Work out the finished part from the listing and answer in its coordinate system (mm). A direction names the side the tool comes from. Coordinates: 2 decimals unless noted, no trailing zeros. Loops run counter-clockwise (first coordinate to the right, second up) from the corner with the lowest first, then second, coordinate; pieces in that order, holes last. Notation, with made-up numbers: M -3,61.25 L 47,61.25 A18 ccw 47,73.25 Z; hole C 37.5,-0.75 d4. An arc over 180 degrees is marked long. Write each question's results on one line, items separated by ' | '.
```python
from build123d import *

# Parameters (mm, degrees)
F0_W     = 4.0655732155
F0_H     = 10
F0_W_2   = 10
F0_H_2   = 4.0655732155
F1_DEPTH = 60
F2_DEPTH = 10
F3_DEPTH = 1


with BuildPart() as f1:
    # F0 (on Top) → F1 (new body)
    with BuildSketch(Plane.XY):
        Polygon((-81.7574552458, 91.9649731191), (-85.0374214202, 91.9649731191), (-85.0374214202, 87.5400633349), (-85.0374214202, 55.211449102), (-85.0374214202, -53.3124324366), (-85.0374214202, -86.6156537372), (-85.0374214202, -90.0350268809), (-80.8175235253, -90.0350268809), (-48.580678454, -90.0350268809), (96.9625785798, -90.0350268809), (96.9625785798, 91.9649731191), align=None)
        Polygon((-33.0721171855, -88.258663221), (-43.0721171855, -88.258663221), (-48.580678454, -88.258663221), (-64.0721171855, -88.258663221), (-64.0721171855, -84.1930900056), (-43.0721171855, -84.1930900056), (-33.0721171855, -84.1930900056), (-33.0721171855, -84.127867623), (-12.0721171855, -84.127867623), (-12.0721171855, -88.258663221), align=None, mode=Mode.SUBTRACT)
        Polygon((-79.1745140415, -38.1238959565), (-79.1745140415, -48.1238959565), (-79.1745140415, -53.3124324366), (-79.1745140415, -69.1238959565), (-83.240087257, -69.1238959565), (-83.240087257, -53.3124324366), (-83.240087257, -48.1238959565), (-83.240087257, -38.1238959565), (-83.3053096395, -38.1238959565), (-83.3053096395, -17.1238959565), (-79.1745140415, -17.1238959565), align=None, mode=Mode.SUBTRACT)
        Polygon((44.9625785798, -83.9851424098), (54.9625785798, -83.9851424098), (60.1511150599, -83.9851424098), (75.9625785798, -83.9851424098), (75.9625785798, -88.0507156253), (60.1511150599, -88.0507156253), (54.9625785798, -88.0507156253), (44.9625785798, -88.0507156253), (44.9625785798, -88.1159380078), (23.9625785798, -88.1159380078), (23.9625785798, -83.9851424098), align=None, mode=Mode.SUBTRACT)
        Polygon((94.8935046063, -37.9912286836), (94.8935046063, -47.9912286836), (94.8935046063, -53.1797651637), (94.8935046063, -68.9912286836), (90.8279313908, -68.9912286836), (90.8279313908, -53.1797651637), (90.8279313908, -47.9912286836), (90.8279313908, -37.9912286836), (90.7627090082, -37.9912286836), (90.7627090082, -16.9912286836), (94.8935046063, -16.9912286836), align=None, mode=Mode.SUBTRACT)
        Polygon((-83.4004647296, 40.0229126219), (-83.4004647296, 50.0229126219), (-83.4004647296, 55.211449102), (-83.4004647296, 71.0229126219), (-79.3348915141, 71.0229126219), (-79.3348915141, 55.211449102), (-79.3348915141, 50.0229126219), (-79.3348915141, 40.0229126219), (-79.2696691316, 40.0229126219), (-79.2696691316, 19.0229126219), (-83.4004647296, 19.0229126219), align=None, mode=Mode.SUBTRACT)
        Polygon((-77.3635556847, 55.211449102), (-77.3635556847, 83.9649731191), (-48.3621415186, 83.9649731191), (61.3571461726, 83.9649731191), (88.6364443153, 83.9649731191), (88.6364443153, -82.0350268809), (-77.3635556847, -82.0350268809), (-77.3635556847, -53.3124324366), align=None, mode=Mode.SUBTRACT)
        Polygon((-33.1736050386, 85.8970538511), (-43.1736050386, 85.8970538511), (-48.3621415186, 85.8970538511), (-64.1736050386, 85.8970538511), (-64.1736050386, 89.9626270666), (-48.3621415186, 89.9626270666), (-43.1736050386, 89.9626270666), (-33.1736050386, 89.9626270666), (-33.1736050386, 90.0278494491), (-12.1736050386, 90.0278494491), (-12.1736050386, 85.8970538511), align=None, mode=Mode.SUBTRACT)
        Polygon((90.7789625961, 39.9640733615), (90.7789625961, 49.9640733615), (90.7789625961, 55.1526098416), (90.7789625961, 70.9640733615), (94.8445358116, 70.9640733615), (94.8445358116, 55.1526098416), (94.8445358116, 49.9640733615), (94.8445358116, 39.9640733615), (94.9097581941, 39.9640733615), (94.9097581941, 18.9640733615), (90.7789625961, 18.9640733615), align=None, mode=Mode.SUBTRACT)
        Polygon((44.9113614697, 89.7324799762), (54.9113614697, 89.7324799762), (61.3571461726, 89.7324799762), (75.9113614697, 89.7324799762), (75.9113614697, 85.6669067607), (61.3571461726, 85.6669067607), (54.9113614697, 85.6669067607), (44.9113614697, 85.6669067607), (44.9113614697, 85.6016843782), (23.9113614697, 85.6016843782), (23.9113614697, 89.7324799762), align=None, mode=Mode.SUBTRACT)
        Polygon((-79.3348915141, 40.0229126219), (-83.4004647296, 40.0229126219), (-83.4004647296, 19.0229126219), (-79.2696691316, 19.0229126219), (-79.2696691316, 40.0229126219), align=None)
        with Locations((-81.3676781219, 45.0229126219)):
            Rectangle(F0_W, F0_H)
        Polygon((-83.4004647296, 55.211449102), (-83.4004647296, 50.0229126219), (-79.3348915141, 50.0229126219), (-79.3348915141, 55.211449102), (-79.3348915141, 71.0229126219), (-83.4004647296, 71.0229126219), align=None)
        Polygon((-48.3621415186, 85.8970538511), (-43.1736050386, 85.8970538511), (-43.1736050386, 89.9626270666), (-48.3621415186, 89.9626270666), (-64.1736050386, 89.9626270666), (-64.1736050386, 85.8970538511), align=None)
        with Locations((-38.1736050386, 87.9298404588)):
            Rectangle(F0_W_2, F0_H_2)
        Polygon((-33.1736050386, 89.9626270666), (-33.1736050386, 85.8970538511), (-12.1736050386, 85.8970538511), (-12.1736050386, 90.0278494491), (-33.1736050386, 90.0278494491), align=None)
        Polygon((44.9113614697, 85.6669067607), (44.9113614697, 89.7324799762), (23.9113614697, 89.7324799762), (23.9113614697, 85.6016843782), (44.9113614697, 85.6016843782), align=None)
        with Locations((49.9113614697, 87.6996933685)):
            Rectangle(F0_W_2, F0_H_2)
        Polygon((61.3571461726, 89.7324799762), (54.9113614697, 89.7324799762), (54.9113614697, 85.6669067607), (61.3571461726, 85.6669067607), (75.9113614697, 85.6669067607), (75.9113614697, 89.7324799762), align=None)
        Polygon((90.7789625961, 55.1526098416), (90.7789625961, 49.9640733615), (94.8445358116, 49.9640733615), (94.8445358116, 55.1526098416), (94.8445358116, 70.9640733615), (90.7789625961, 70.9640733615), align=None)
        with Locations((92.8117492038, 44.9640733615)):
            Rectangle(F0_W, F0_H)
        Polygon((94.8445358116, 39.9640733615), (90.7789625961, 39.9640733615), (90.7789625961, 18.9640733615), (94.9097581941, 18.9640733615), (94.9097581941, 39.9640733615), align=None)
        Polygon((90.8279313908, -37.9912286836), (94.8935046063, -37.9912286836), (94.8935046063, -16.9912286836), (90.7627090082, -16.9912286836), (90.7627090082, -37.9912286836), align=None)
        with Locations((92.8607179985, -42.9912286836)):
            Rectangle(F0_W, F0_H)
        Polygon((94.8935046063, -53.1797651637), (94.8935046063, -47.9912286836), (90.8279313908, -47.9912286836), (90.8279313908, -53.1797651637), (90.8279313908, -68.9912286836), (94.8935046063, -68.9912286836), align=None)
        Polygon((60.1511150599, -83.9851424098), (54.9625785798, -83.9851424098), (54.9625785798, -88.0507156253), (60.1511150599, -88.0507156253), (75.9625785798, -88.0507156253), (75.9625785798, -83.9851424098), align=None)
        with Locations((49.9625785798, -86.0179290175)):
            Rectangle(F0_W_2, F0_H_2)
        Polygon((44.9625785798, -88.0507156253), (44.9625785798, -83.9851424098), (23.9625785798, -83.9851424098), (23.9625785798, -88.1159380078), (44.9625785798, -88.1159380078), align=None)
        Polygon((-33.0721171855, -84.1930900056), (-33.0721171855, -88.258663221), (-12.0721171855, -88.258663221), (-12.0721171855, -84.127867623), (-33.0721171855, -84.127867623), align=None)
        with Locations((-38.0721171855, -86.2258766133)):
            Rectangle(F0_W_2, F0_H_2)
        Polygon((-48.580678454, -88.258663221), (-43.0721171855, -88.258663221), (-43.0721171855, -84.1930900056), (-64.0721171855, -84.1930900056), (-64.0721171855, -88.258663221), align=None)
        Polygon((-79.1745140415, -53.3124324366), (-79.1745140415, -48.1238959565), (-83.240087257, -48.1238959565), (-83.240087257, -53.3124324366), (-83.240087257, -69.1238959565), (-79.1745140415, -69.1238959565), align=None)
        with Locations((-81.2073006492, -43.1238959565)):
            Rectangle(F0_W, F0_H)
        Polygon((-83.240087257, -38.1238959565), (-79.1745140415, -38.1238959565), (-79.1745140415, -17.1238959565), (-83.3053096395, -17.1238959565), (-83.3053096395, -38.1238959565), align=None)
    extrude(amount=-F1_DEPTH)

    # F0 (on Top) → F2 (cut)
    with BuildSketch(Plane.XY):
        Polygon((-83.4004647296, 55.211449102), (-83.4004647296, 50.0229126219), (-79.3348915141, 50.0229126219), (-79.3348915141, 55.211449102), (-79.3348915141, 71.0229126219), (-83.4004647296, 71.0229126219), align=None)
        Polygon((-79.3348915141, 40.0229126219), (-83.4004647296, 40.0229126219), (-83.4004647296, 19.0229126219), (-79.2696691316, 19.0229126219), (-79.2696691316, 40.0229126219), align=None)
        Polygon((90.7789625961, 55.1526098416), (90.7789625961, 49.9640733615), (94.8445358116, 49.9640733615), (94.8445358116, 55.1526098416), (94.8445358116, 70.9640733615), (90.7789625961, 70.9640733615), align=None)
        Polygon((94.8445358116, 39.9640733615), (90.7789625961, 39.9640733615), (90.7789625961, 18.9640733615), (94.9097581941, 18.9640733615), (94.9097581941, 39.9640733615), align=None)
        Polygon((-83.240087257, -38.1238959565), (-79.1745140415, -38.1238959565), (-79.1745140415, -17.1238959565), (-83.3053096395, -17.1238959565), (-83.3053096395, -38.1238959565), align=None)
        Polygon((-79.1745140415, -53.3124324366), (-79.1745140415, -48.1238959565), (-83.240087257, -48.1238959565), (-83.240087257, -53.3124324366), (-83.240087257, -69.1238959565), (-79.1745140415, -69.1238959565), align=None)
        Polygon((94.8935046063, -53.1797651637), (94.8935046063, -47.9912286836), (90.8279313908, -47.9912286836), (90.8279313908, -53.1797651637), (90.8279313908, -68.9912286836), (94.8935046063, -68.9912286836), align=None)
        Polygon((90.8279313908, -37.9912286836), (94.8935046063, -37.9912286836), (94.8935046063, -16.9912286836), (90.7627090082, -16.9912286836), (90.7627090082, -37.9912286836), align=None)
        Polygon((61.3571461726, 89.7324799762), (54.9113614697, 89.7324799762), (54.9113614697, 85.6669067607), (61.3571461726, 85.6669067607), (75.9113614697, 85.6669067607), (75.9113614697, 89.7324799762), align=None)
        Polygon((44.9113614697, 85.6669067607), (44.9113614697, 89.7324799762), (23.9113614697, 89.7324799762), (23.9113614697, 85.6016843782), (44.9113614697, 85.6016843782), align=None)
        Polygon((-33.1736050386, 89.9626270666), (-33.1736050386, 85.8970538511), (-12.1736050386, 85.8970538511), (-12.1736050386, 90.0278494491), (-33.1736050386, 90.0278494491), align=None)
        Polygon((-48.3621415186, 85.8970538511), (-43.1736050386, 85.8970538511), (-43.1736050386, 89.9626270666), (-48.3621415186, 89.9626270666), (-64.1736050386, 89.9626270666), (-64.1736050386, 85.8970538511), align=None)
    extrude(amount=-F2_DEPTH, mode=Mode.SUBTRACT)

    # F0 (on Top) → F3 (cut)
    with BuildSketch(Plane.XY):
        with Locations((-81.3676781219, 45.0229126219)):
            Rectangle(F0_W, F0_H)
        with Locations((-81.2073006492, -43.1238959565)):
            Rectangle(F0_W, F0_H)
        with Locations((92.8607179985, -42.9912286836)):
            Rectangle(F0_W, F0_H)
        with Locations((92.8117492038, 44.9640733615)):
            Rectangle(F0_W, F0_H)
        with Locations((49.9113614697, 87.6996933685)):
            Rectangle(F0_W_2, F0_H_2)
        with Locations((-38.1736050386, 87.9298404588)):
            Rectangle(F0_W_2, F0_H_2)
        with Locations((-38.0721171855, -86.2258766133)):
            Rectangle(F0_W_2, F0_H_2)
        with Locations((49.9625785798, -86.0179290175)):
            Rectangle(F0_W_2, F0_H_2)
    extrude(amount=-F3_DEPTH, mode=Mode.SUBTRACT)


solid = f1.part
```
1) Find section A-A, the plane x = -22. Give the vertices of the cut face in (y, z), and give its area (3 significant figures).
Check result:
outline: M -90.04,-60 L -82.04,-60 L -82.04,0 L -90.04,0 Z; M 83.96,-60 L 91.96,-60 L 91.96,0 L 90.03,0 L 90.03,-10 L 85.9,-10 L 85.9,0 L 83.96,0 Z | area: 919 mm^2
2) Given pin 1 Ø4.5 at (x, y) = (92.5, 56) entering from +Z; pin 2 Ø1.2 at (x, y) = (92, 43) entering from +Z; pin 3 Ø2 at (x, y) = (-81.5, -28) entering from +Z, each flat-ended and moving along its own axis, determine where each tip first touches the part or whether it passes through.
Check result:
pin 1: z = 0 | pin 2: z = -1 | pin 3: z = -10
3) Find section D-D, the plane x = -58.5. Give the vertices of the cut face in (y, z).
Check result:
outline: M -90.04,-60 L -82.04,-60 L -82.04,0 L -90.04,0 Z; M 83.96,-60 L 91.96,-60 L 91.96,0 L 89.96,0 L 89.96,-10 L 85.9,-10 L 85.9,0 L 83.96,0 Z
4) Find section B-B, the plane y = 79. Give the vertices of the cut face in (x, z).
Check result:
outline: M -85.04,-60 L -77.36,-60 L -77.36,0 L -85.04,0 Z; M 88.64,-60 L 96.96,-60 L 96.96,0 L 88.64,0 Z
5) Find section C-C, the plane z = -26. Give the vertices of the cut face in (x, y).
Check result:
outline: M -85.04,-90.04 L 96.96,-90.04 L 96.96,91.96 L -85.04,91.96 Z; hole M -77.36,-82.04 L 88.64,-82.04 L 88.64,83.96 L -77.36,83.96 Z
6) Straight lines are drawn through the part: probe 1 along X at (y, z) = (-59, -4.5); probe 2 along Y at (x, z) = (39.5, -34); probe 3 along X at (y, z) = (-44, -29). For each, find the intervals that lie inside material, in ascending order. Write a range as [from, to].
Check result:
probe 1: [-85.04, -83.24], [-79.17, -77.36], [88.64, 90.83], [94.89, 96.96] | probe 2: [-90.04, -82.04], [83.96, 91.96] | probe 3: [-85.04, -77.36], [88.64, 96.96]
7) For a pull along Z with two mould halves and no side action, classify faces 1 (the face through (93, 30, -10)), 2 (the face through (93, 39.964, -6)) as released by +Z, released by -Z, zero draft, split by the parting line, or undercut.
Check result:
face 1: released by +Z | face 2: zero draft
8) Which of the six approach directions +Z, -Z, +X, -X, +Y, -Y give full straight-line access (tool end or side, diameter ignored) to faces 3 (the face through (94.894, -43.4, -0.5)), 4 (the face through (88.636, 2, -30))?
Check result:
face 3: +Z | face 4: +Z, -Z
